```python
from build123d import *

# Parameters (mm, degrees)
F0_W      = 64.7
F0_H      = 138.7
F1_DEPTH  = 2
F1_FACE_W = 64.7
F1_FACE_H = 138.7
F2_DEPTH  = 1.5
F3_W      = 64.5
F3_H      = 116.084408
F4_DEPTH  = 43.240232


with BuildPart() as f1:
    # F0 (on Front) → F1 (new body)
    with BuildSketch(Plane.XZ):
        Rectangle(F0_W, F0_H)
    extrude(amount=F1_DEPTH)

    # F1_face (on face) → F2 (cut)
    with BuildSketch(Plane(origin=(0, 0, 0), x_dir=(1, 0, 0), z_dir=(0, 1, 0))):
        Rectangle(F1_FACE_W, F1_FACE_H)
    extrude(amount=-F2_DEPTH, mode=Mode.SUBTRACT)

    # F3 (on Front) → F4 (cut)
    with BuildSketch(Plane.XZ):
        Rectangle(F3_W, F3_H)
    extrude(amount=F4_DEPTH, mode=Mode.SUBTRACT)


solid = f1.part
```
Check sheet for the modelled part. Datum: model origin and axes. Units: mm. Round coordinates to 2 decimals unless told otherwise and drop trailing zeros. Loops run counter-clockwise (first coordinate to the right, second up) from the corner with the lowest first, then second, coordinate; pieces in that order, holes last. Notation, with made-up numbers: M 82.5,88.5 L 128.5,88.5 A20 cw 128.5,127.5 Z; hole C -3.75,63 d11. An arc over 180 degrees is marked long. Answer as a JSON object with one key per item and string values.
1. Scan line: line 1 (Z direction, x = 2.5, y = -1.9). Record every from-to range of solid material in increasing order.
Reply:
{"line 1": "z = -69.35 to -58.04, 58.04 to 69.35"}
2. Section check B-B (x = 0.5). Record the boundary of the cut face in (y, z), plus the area to 3 significant figures.
Reply:
{"outline": "M -2,-69.35 L -1.5,-69.35 L -1.5,-58.04 L -2,-58.04 Z; M -2,58.04 L -1.5,58.04 L -1.5,69.35 L -2,69.35 Z", "area": "11.3 mm²"}
3. Section check A-A (z = -30). Record the boundary of the cut face in (x, y).
Reply:
{"outline": "M -32.35,-2 L -32.25,-2 L -32.25,-1.5 L -32.35,-1.5 Z; M 32.25,-2 L 32.35,-2 L 32.35,-1.5 L 32.25,-1.5 Z"}
4. Section check C-C (y = -1.6). Record the boundary of the cut face in (x, z), plus the area to 3 significant figures.
Reply:
{"outline": "M -32.35,-69.35 L 32.35,-69.35 L 32.35,69.35 L -32.35,69.35 Z; hole M -32.25,-58.04 L 32.25,-58.04 L 32.25,58.04 L -32.25,58.04 Z", "area": "1,490 mm²"}
